Here's how the part is built. I have some questions about the finished solid (model axes, mm). Round coordinates to 2 decimals unless told otherwise and drop trailing zeros. Loops run counter-clockwise (first coordinate to the right, second up) from the corner with the lowest first, then second, coordinate; pieces in that order, holes last. Notation, with made-up numbers: M -18.5,63 L -11.5,63 A32 ccw -11.5,90 Z; hole C -34.5,-38.5 d2. An arc over 180 degrees is marked long. Answer as a JSON object with one key per item and string values.
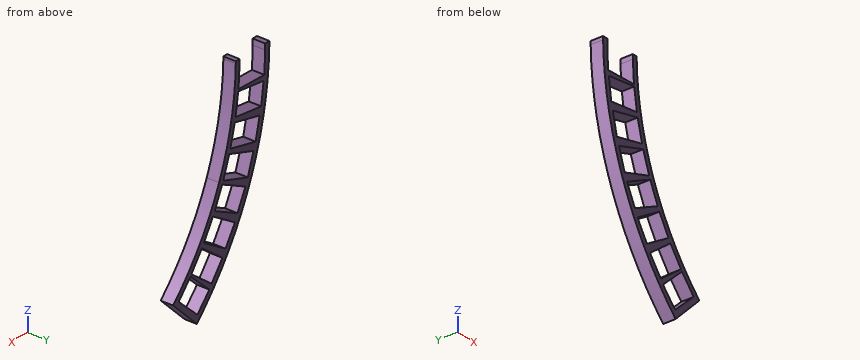
from build123d import *

# Parameters (mm, degrees)
BOSS_EXTRUDE1_DEPTH = 12


with BuildPart() as part:
    # Sketch1 → Boss-Extrude1 (new body)
    with BuildSketch(Plane(origin=(0, 0, 0), x_dir=(1, 0, 0), z_dir=(0, 1, 0))):
        with BuildLine():
            Line((-208.730747898, 208.730747898), (-180.446460839, 180.446460839))
            ThreePointArc((-180.446460839, 180.446460839), (-211.871169585, 142.237594702), (-235.332727793, 98.683202756))
            ThreePointArc((-235.332727793, 98.683202756), (-249.691614544, 52.678245772), (-255.14471115, 4.794037172))
            Line((-255.14471115, 4.794037172), (-255.14471115, 2.779626551))
            Line((-255.14471115, 2.779626551), (-259.672052343, 2.779626551))
            Line((-259.672052343, 2.779626551), (-259.672052343, 7.204875095))
            Line((-259.672052343, 7.204875095), (-258.35063673, 28.168690687))
            Line((-258.35063673, 28.168690687), (-289.227344139, 29.411556091))
            Line((-289.227344139, 29.411556091), (-290.170172115, 8.432501391))
            Line((-290.170172115, 8.432501391), (-290.170172115, 2.779626551))
            Line((-290.170172115, 2.779626551), (-295.127762341, 2.779626551))
            Line((-295.127762341, 2.779626551), (-295.127762341, 6.054265565))
            ThreePointArc((-295.127762341, 6.054265565), (-271.547028538, 115.755179272), (-208.730747898, 208.730747898))
        make_face()
        Polygon((-288.286547304, 34.069084362), (-258.033222279, 30.008925637), (-254.767009525, 50.758854735), (-285.491553173, 54.882253531), align=None, mode=Mode.SUBTRACT)
        Polygon((-283.612878523, 61.915838046), (-253.89939669, 54.933619681), (-248.631031599, 75.267631401), (-278.809043274, 82.359007245), align=None, mode=Mode.SUBTRACT)
        Polygon((-276.255921554, 89.176800074), (-247.361344598, 79.340855863), (-240.142390382, 99.066838813), (-269.488694715, 109.056554622), align=None, mode=Mode.SUBTRACT)
        Polygon((-229.967759139, 120.819849226), (-238.977493449, 101.844802692), (-266.671759318, 115.77418308), (-257.235727442, 134.534814797), align=None, mode=Mode.SUBTRACT)
        Polygon((-217.141868251, 142.590375773), (-227.952465343, 124.580414811), (-254.16244031, 141.134484167), (-242.948393328, 158.889628499), align=None, mode=Mode.SUBTRACT)
        Polygon((-202.261755682, 163.008777697), (-214.772333152, 146.135332444), (-239.248466479, 165.159498585), (-226.362501502, 181.741172494), align=None, mode=Mode.SUBTRACT)
        Polygon((-187.145427565, 180.161244264), (-201.171686006, 164.525011421), (-223.699930588, 185.676700973), (-209.397447264, 201.053587246), align=None, mode=Mode.SUBTRACT)
    extrude(amount=BOSS_EXTRUDE1_DEPTH)


solid = part.part
Item 1: I want a section at B-B on z = -59. List the corners of the cut face in (x, y) for me, plus the area to 3 significant figures.
Solution:
{"outline": "M -289.23,0 L -271.2,0 L -271.2,12 L -289.23,12 Z; M -252.85,0 L -248.27,0 L -248.27,12 L -252.85,12 Z", "area": "271 mm2"}
Item 2: I want a section at D-D on z = -188.5. List the corners of the cut face in (x, y) for me.
Solution:
{"outline": "M -227.17,0 L -221.07,0 L -221.07,12 L -227.17,12 Z; M -196.03,0 L -188.5,0 L -188.5,12 L -196.03,12 Z"}
Item 3: For P1, Ø3, axis at x = -221, y = 4.5, coming from the +Z side; P2, Ø5, axis at y = 3, z = -80, coming from the +X side; P3, Ø5, axis at y = 6, z = -100, coming from the -X side, each with a flat end and sliding along its axis, tell me the tip position at first contact or that it passes through.
Solution:
{"P1": "stops at z = -124.96", "P2": "stops at x = -241.48", "P3": "stops at x = -278.62"}
Item 4: I want a section at A-A on z = -167.5. List the corners of the cut face in (x, y) for me.
Solution:
{"outline": "M -243.07,0 L -237.43,0 L -237.43,12 L -243.07,12 Z; M -208.04,0 L -204.34,0 L -204.34,12 L -208.04,12 Z; M -198.5,0 L -192.52,0 L -192.52,12 L -198.5,12 Z"}
Item 5: I want a section at C-C on y = 4. Count the separate pieces of the cut face and the enclosed holes in it, plus the area to 3 significant figures.
Solution:
{"separate pieces": "1", "enclosed holes": "7", "area": "3,210 mm2"}
Item 6: If I drill on L1, parallel to Z at x = -210.5, y = 9.5; L2, parallel to Z at x = -226.5, y = 9; L3, parallel to Z at x = -235, y = 11, over which ranges is the centre line in solid material (lowest first)? Write a range as from..to.
Solution:
{"L1": "z = -206.95..-199.87, -173.28..-169.41, -151.9..-144.26", "L2": "z = -189.3..-181.56, -155.25..-148.5, -127..-117.55", "L3": "z = -178.64..-170.63, -161.86..-153.87, -129.03..-123.35, -110.22..-99.47"}
